Geometry check sheet. Reference: the model listing, model coordinates, mm. A direction names the side the tool comes from. Coordinates: 2 decimals unless noted, no trailing zeros. Write each loop counter-clockwise with the first axis right and the second up, starting at its lowest first coordinate (ties: lowest second). Pieces come first, ordered by that corner, then holes. Notation, with made-up numbers: (0.5, 3.25) - (46.5, 3.25) arc R30 cw to (46.5, 36.25) - close; hole circle Ø3 at (55.5, -32). An arc over 180 degrees is marked (long way). Answer as a JSON object with one key per item and string values. Group by question number.
from build123d import *

# Parameters (mm, degrees)
SKETCH_1_W          = 280
SKETCH_1_H          = 200
SKETCH_1_R          = 85
EXTRUDE_1_DEPTH     = 3
SKETCH_1_4_R        = 85
SKETCH_1_4_R_2      = 2
SKETCH_1_4_R_3      = 75
EXTRUDE_3_DEPTH     = 5
SKETCH_2_W          = 44
SKETCH_2_H          = 44
SKETCH_2_W_2        = 40
SKETCH_2_H_2        = 40
EXTRUDE_4_DEPTH     = 50
SKETCH_3_R          = 1
CUT_EXTRUDE_1_DEPTH = 50


with BuildPart() as part:
    # Sketch 1 → Extrude 1 (new body)
    with BuildSketch(Plane(origin=(0, 0, 0), x_dir=(1, 0, 0), z_dir=(0, 1, 0))):
        Rectangle(SKETCH_1_W, SKETCH_1_H)
        with Locations(Location((-50, 0, 0), (0, 0, 270))):
            Circle(SKETCH_1_R, mode=Mode.SUBTRACT)
    extrude(amount=EXTRUDE_1_DEPTH)

    # Sketch 1_4 → Extrude 3 (add)
    with BuildSketch(Plane(origin=(0, 0, 0), x_dir=(1, 0, 0), z_dir=(0, 1, 0))):
        with Locations(Location((-50, 0, 0), (0, 0, 270))):
            Circle(SKETCH_1_4_R)
        with Locations(Location((-130, 0, 0), (0, 0, 270))):
            Circle(SKETCH_1_4_R_2, mode=Mode.SUBTRACT)
        with Locations(Location((30, 0, 0), (0, 0, 270))):
            Circle(SKETCH_1_4_R_2, mode=Mode.SUBTRACT)
        with Locations(Location((-50, 0, 0), (0, 0, 270))):
            Circle(SKETCH_1_4_R_3, mode=Mode.SUBTRACT)
        with Locations(Location((-50, 80, 0), (0, 0, 270))):
            Circle(SKETCH_1_4_R_2, mode=Mode.SUBTRACT)
        with Locations(Location((-50, -80, 0), (0, 0, 270))):
            Circle(SKETCH_1_4_R_2, mode=Mode.SUBTRACT)
    extrude(amount=EXTRUDE_3_DEPTH)

    # Sketch 2 → Extrude 4 (add)
    with BuildSketch(Plane(origin=(0, 3, 0), x_dir=(1, 0, 0), z_dir=(0, 1, 0))):
        with Locations((72.175056864, 0.848639526)):
            Rectangle(SKETCH_2_W, SKETCH_2_H)
        with Locations((72.175056864, 0.848639526)):
            Rectangle(SKETCH_2_W_2, SKETCH_2_H_2, mode=Mode.SUBTRACT)
    extrude(amount=EXTRUDE_4_DEPTH)

    # Sketch 3 → Cut-Extrude 1 (cut)
    with BuildSketch(Plane(origin=(0, 3, 0), x_dir=(1, 0, 0), z_dir=(0, 1, 0))):
        with Locations(Location((72.175056864, 0.848639526, 0), (0, 0, 270))):
            Circle(SKETCH_3_R)
    extrude(amount=-CUT_EXTRUDE_1_DEPTH, mode=Mode.SUBTRACT)


solid = part.part
(1) Set-up check for faces 1 (the face through (72, 28, 19.151)), 2 (the face through (70, 53, 20)), 3 (the face through (-125.2, 5, -0.4)): record each of +Z, -Z, +X, -X, +Y, -Y from which the full face is reachable in a straight line by a thin tool's end or side.
(2) Gauge pin test, flat ends, axial feed: pin 1 (8 mm diameter, centred on y = 6, z = -38.5, fed in from +X); pin 2 (5 mm diameter, centred on y = 8, z = -4, fed in from -X); pin 3 (20 mm diameter, centred on y = 37, z = 4.5, fed in from +X); pin 4 (13 mm diameter, centred on x = 76.5, y = 25.5, fed in from -Z). Record the tip position at first contact, or that the pin passes through.
(3) Section check D-D (x = -26.5). Record the cut outline in (y, z).
(4) Section check B-B (y = 27). Record the cut outline in (x, z).
(5) Material ranges on L1, parallel to X at y = 3.5, z = -10.5; L2, parallel to X at y = 35.5, z = -20.5; L3, parallel to X at y = 2, z = 0, recorded low to high. Write a range as [from, to].
(6) Section check C-C (z = -88). Record the cut outline in (x, y), and give its area (3 significant figures).
(7) Section check A-A (x = -56.5). Record the cut outline in (y, z), and give its area (3 significant figures).
(8) Draft check along X on faces 4 (the face through (94.175, 28, -1)), 5 (the face through (72, 28, -22.849)), 6 (the face through (72, 28, -20.849)). Enter one of: +X half, -X half, draft (parallel to the pull), parting line (faces both ways), or undercut.
Conclusion:
{
 "1": {"face 1": "+Y", "face 2": "+Z, -Z, +X, -X, +Y", "face 3": "+Z, -Z, -X, +Y"},
 "2": {"pin 1": "stops at x = 140", "pin 2": "stops at x = 50.18", "pin 3": "stops at x = 94.18", "pin 4": "stops at z = -22.85"},
 "3": {"outline": "(0, -100) - (3, -100) - (3, -81.69) - (5, -81.69) - (5, -71.22) - (0, -71.22) - close; (0, 71.22) - (5, 71.22) - (5, 81.69) - (3, 81.69) - (3, 100) - (0, 100) - close"},
 "4": {"outline": "(50.18, -22.85) - (94.18, -22.85) - (94.18, 21.15) - (50.18, 21.15) - close; hole (52.18, -20.85) - (92.18, -20.85) - (92.18, 19.15) - (52.18, 19.15) - close"},
 "5": {"L1": "x = [-134.35, -124.26], [24.26, 34.35], [50.18, 52.18], [92.18, 94.18]", "L2": "x = [50.18, 52.18], [92.18, 94.18]", "L3": "x = [-140, -132], [-128, -125], [25, 28], [32, 71.65], [72.7, 140]"},
 "6": {"outline": "(-140, 0) - (140, 0) - (140, 3) - (-140, 3) - close", "area": "840 mm^2"},
 "7": {"outline": "(0, -100) - (3, -100) - (3, -84.75) - (5, -84.75) - (5, -74.72) - (0, -74.72) - close; (0, 74.72) - (5, 74.72) - (5, 84.75) - (3, 84.75) - (3, 100) - (0, 100) - close", "area": "192 mm^2"},
 "8": {"face 4": "+X half", "face 5": "draft", "face 6": "undercut"}
}
